The listing builds one solid part. Answer for the finished solid, in the listing's coordinates (mm). Face numbers are marked on the shaded views. Coordinates: 2 decimals unless noted, no trailing zeros. Order: outer loops, then holes, each group sorted by start corner. A loop starts at its lowest first (then second) coordinate and runs counter-clockwise, first axis right, second up. Notation, with made-up numbers: (-11, 20.25) -> (25, 20.25) arc R24 cw to (25, 46.25) -> close; hole circle Ø2 at (53.5, 10). An arc over 180 degrees is marked (long way). Put each result on its own line as item: value. Start each with the question number.
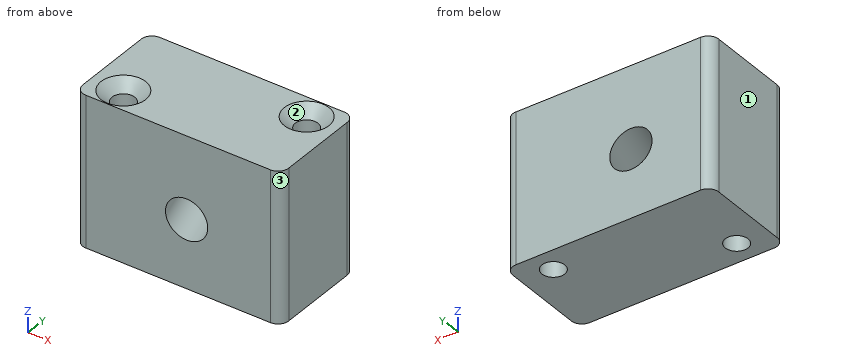
```python
from build123d import *

# Parameters (mm, degrees)
BOSS_EXTRUDE1_DEPTH                             = 17.45
CSK_FOR_M5_FLAT_HEAD_MACHINE_SCREW1_D           = 5.3
CSK_FOR_M5_FLAT_HEAD_MACHINE_SCREW1_CSINK_D     = 10.4
CSK_FOR_M5_FLAT_HEAD_MACHINE_SCREW1_CSINK_ANGLE = 90
SKETCH24_W                                      = 4.699
SKETCH24_H                                      = 43.607186054


with BuildPart() as part:
    # Sketch1 → Boss-Extrude1 (new body, symmetric)
    with BuildSketch(Plane.XY):
        with BuildLine():
            Line((-21.45, -11.95), (21.45, -11.95))
            ThreePointArc((21.45, -11.95), (23.217766953, -11.217766953), (23.95, -9.45))
            Line((23.95, -9.45), (23.95, 9.45))
            ThreePointArc((23.95, 9.45), (23.217766953, 11.217766953), (21.45, 11.95))
            Line((21.45, 11.95), (-21.45, 11.95))
            ThreePointArc((-21.45, 11.95), (-23.217766953, 11.217766953), (-23.95, 9.45))
            Line((-23.95, 9.45), (-23.95, -9.45))
            ThreePointArc((-23.95, -9.45), (-23.217766953, -11.217766953), (-21.45, -11.95))
        make_face()
    extrude(amount=BOSS_EXTRUDE1_DEPTH, both=True)

    # CSK for M5 Flat Head Machine Screw1 (through all)
    with Locations(Plane.XY.offset(17.45)):
        with Locations((-16.605361405, -6.552011076), (16.605361405, 6.552011076)):
            CounterSinkHole(CSK_FOR_M5_FLAT_HEAD_MACHINE_SCREW1_D / 2, CSK_FOR_M5_FLAT_HEAD_MACHINE_SCREW1_CSINK_D / 2, counter_sink_angle=CSK_FOR_M5_FLAT_HEAD_MACHINE_SCREW1_CSINK_ANGLE)

    # Sketch24 → Cut-Revolve2 (revolve, cut)
    with BuildSketch(Plane(origin=(-1.518528381, -0.464260717, 0), x_dir=(0, 0, -1), z_dir=(0.956304756, 0.292371705, 0))):
        with Locations((3.9795, -0.045167625)):
            Rectangle(SKETCH24_W, SKETCH24_H)
    revolve(axis=Axis((-7.880076307, 20.343424977, -1.63), (0.292371705, -0.956304756, 0)), mode=Mode.SUBTRACT)


solid = part.part
```
(1) The part is cut by section A-A on z = -10.5. Determine the outline of the cut face in (x, y), plus the area to 3 significant figures.
(2) This flat-tipped pin is pushed along its axis until it touches: P1, Ø4, axis at x = 0, z = -4, coming from the -Y side. Where does it stop, or does it pass through?
(3) For a pull along X with two mould halves and no side action, classify the marked faces 1, 2 and 3 as released by +X, released by -X, zero draft, split by the parting line, or undercut.
(4) The part is cut by section B-B on y = -5.75. Count the separate pieces of the cut face and the enclosed holes in it, plus the area to 3 significant figures.
(5) Find the intervals of material crossed by L1, parallel to X at y = -8.25, z = -1; L2, parallel to Y at x = -17.5, z = -12; L3, parallel to Z at x = -6, y = -0.5, in increasing order.
Worked out:
1. outline: (-23.95, -9.45) arc R2.5 ccw to (-21.45, -11.95) -> (21.45, -11.95) arc R2.5 ccw to (23.95, -9.45) -> (23.95, 9.45) arc R2.5 ccw to (21.45, 11.95) -> (-21.45, 11.95) arc R2.5 ccw to (-23.95, 9.45) -> close; hole circle Ø5.3 at (-16.61, -6.55); hole circle Ø5.3 at (16.61, 6.55)
1. area: 1,100 mm2
2. P1: y = -11.95
3. face 1: released by -X
3. face 2: undercut
3. face 3: released by +X
4. separate pieces: 2
4. enclosed holes: 1
4. area: 1,420 mm2
5. L1: -23.95 to -18.64, -14.57 to -4.01, 5.73 to 23.95
5. L2: -11.95 to -9.05, -4.06 to 11.95
5. L3: -17.45 to -3.53, 0.27 to 17.45
